The model under review builds one solid part; all positions refer to its coordinate system, in mm. A direction names the side the tool comes from. Round coordinates to 2 decimals unless told otherwise and drop trailing zeros. Write each loop counter-clockwise with the first axis right and the second up, starting at its lowest first coordinate (ties: lowest second). Pieces come first, ordered by that corner, then holes. Notation, with made-up numbers: M 50.25,4 L 80.25,4 A9 ccw 80.25,18 Z; hole C -16,88.25 d6. An arc over 180 degrees is marked long. One line per item, written item: value. Start each with the question number.
1) Mouldability with a two-part tool opening along Y and no side actions: class faces 1 (the face through (-9, 42, 5)), 2 (the face through (0, 57, 0)), 3 (the face through (-10, 42, -3)), 4 (the face through (-2.309, 49.605, 10.755)) as +Y half, -Y half, draft (parallel to the pull), parting line (faces both ways), or undercut.
2) Tool access review of faces 5 (the face through (-6.1, 42, 8.4)), 6 (the face through (0, 37, 0)), 7 (the face through (6.1, 42, 8.4)): name each direction out of +Z, -Z, +X, -X, +Y, -Y from which nothing blocks a thin tool from reaching the whole face with its end or side.
3) Wall thickness on probe 1 along Z at (x, y) = (0, 24.5); probe 2 along Y at (x, z) = (6, -6); probe 3 along Y at (x, z) = (7, 12): over which ranges is each line inside the solid? List them lowest first.
4) For P1, Ø6, axis at x = -1.5, z = 3.5, coming from the -Y side; P2, Ø8, axis at y = 10, z = 5, coming from the -X side; P3, Ø1, axis at x = -11.5, z = -4, coming from the +Y side, all flat-tipped, find the tip position at first contact; note any pin that passes through.
5) Take a section at B-B, the plane y = 38. Write out the cut boundary in (x, z).
6) Take a section at A-A, the plane y = 9. Write out the cut boundary in (x, z).
from build123d import *

# Parameters (mm, degrees)
CHAMFER1_SIZE       = 1
FILLET1_SIZE        = 1
SKETCH2_R           = 1
BOSS_EXTRUDE1_DEPTH = 15
CIRPATTERN1_COUNT   = 15


with BuildPart() as part:
    # Sketch1 → Revolve1 (revolve)
    with BuildSketch(Plane.XY, mode=Mode.PRIVATE) as revolve1_sk:
        Polygon((15, 0), (15, 40), (10, 40), (10, 57), (0, 57), (0, 37), (12, 37), (12, 0), align=None)
    revolve(revolve1_sk.sketch.rotate(Axis((0, 57, 0), (0, -1, 0)), 180), axis=Axis((0, 57, 0), (0, -1, 0)))

    # Chamfer1
    chamfer1_edges = [part.edges().sort_by_distance(p)[0] for p in [
        (12, 0, 0),
        (10, 40, 0),
        (15, 40, 0),
    ]]
    chamfer(chamfer1_edges, length=CHAMFER1_SIZE)

    # Fillet1
    # a fillet whose section is not a circle: 1 mm, written as the material it takes off along each edge
    with BuildSketch(Plane(origin=(0, 0, 0), x_dir=(-1, 0, 0), z_dir=(0, 0, 1))) as fillet1_piece_1:
        with BuildLine():
            add(Edge.make_bspline([(15, -FILLET1_SIZE), (15, -FILLET1_SIZE * 0.831801948466), (15, -FILLET1_SIZE * 0.663603896932), (15 - FILLET1_SIZE * 0.0716919198361, -FILLET1_SIZE * 0.292893218813), (15 - FILLET1_SIZE * 0.292893218813, -FILLET1_SIZE * 0.0716919198361), (15 - FILLET1_SIZE * 0.663603896932, 0), (15 - FILLET1_SIZE * 0.831801948466, 0), (15 - FILLET1_SIZE, 0)], knots=[0, 0, 0, 0, 0, 0, 0.5, 0.5, 1, 1, 1, 1, 1, 1], degree=5))
            Line((15 - FILLET1_SIZE, 0), (15, 0))
            Line((15, 0), (15, -FILLET1_SIZE))
        make_face()
    revolve(axis=Axis((0, 0, 0), (0, -1, 0)), mode=Mode.SUBTRACT)

    # Sketch2 → Boss-Extrude1 (add)
    with BuildSketch(Plane(origin=(0, 57, 0), x_dir=(1, 0, 0), z_dir=(0, 1, 0))):
        with Locations((0, 10)):
            Circle(SKETCH2_R)
    boss_extrude1 = extrude(amount=-BOSS_EXTRUDE1_DEPTH)

    # CirPattern1: Boss-Extrude1 ×15 about axis
    cirpattern1_axis = Axis((0, 0, 0), (0, 1, 0))
    for i in range(1, CIRPATTERN1_COUNT):
        add(boss_extrude1.rotate(cirpattern1_axis, i * 360 / CIRPATTERN1_COUNT))


solid = part.part
Checked values:
1. face 1: undercut
1. face 2: +Y half
1. face 3: undercut
1. face 4: draft
2. face 5: +Z, -X
2. face 6: -Y
2. face 7: +Z, +X
3. probe 1: z = -15 to -12, 12 to 15
3. probe 2: y = 37 to 57
3. probe 3: y = 0 to 40
4. P1: stops at y = 37
4. P2: stops at x = -14.97
4. P3: stops at y = 40
5. outline: C 0,0 d30
6. outline: C 0,0 d30; hole C 0,0 d24
